Part model, mm, in its own coordinate system. A direction names the side the tool comes from. Round coordinates to 2 decimals unless told otherwise and drop trailing zeros. Loops run counter-clockwise (first coordinate to the right, second up) from the corner with the lowest first, then second, coordinate; pieces in that order, holes last. Notation, with made-up numbers: (40, 51) - (78, 51) arc R20 ccw to (78, 90) - close; hole circle Ø8 at (-4.5, 46.25). An arc over 180 degrees is marked (long way). Write each question's results on one line, items separated by ' | '. Start each with the question number.
(1) Cut at A-A, the plane z = 10. List the corners of the cut face in (x, y), then the cut area to 3 significant figures.
(2) Cut at D-D, the plane x = 2. List the corners of the cut face in (y, z), then the cut area to 3 significant figures.
(3) Mould opens along X. For faces 1 (the face through (0.14, -7.57, 19.4)), 2 (the face through (-1.06, 2.57, -18.48)), 3 (the face through (-10, -7.4, -5.8)) say: released by +X, released by -X, zero draft, split by the parting line, or undercut.
(4) Drill centre lines: L1, parallel to X at y = -9.4, z = -10; L2, parallel to Y at x = -3.5, z = 14. Where is each one in solid material? Low to high.
(5) Tool access for faces 4 (the face through (0, 3, -17)), 5 (the face through (0.1, 10, -19.5)): list every direction of +Z, -Z, +X, -X, +Y, -Y with a clear straight run to the whole face (end or side of a thin tool).
(6) Cut at C-C, the plane x = -3.25. List the corners of the cut face in (y, z).
(7) Cut at B-B, the plane y = 0. List the corners of the cut face in (x, z), then the cut area to 3 significant figures.
(8) Flat gauge pins, fed straight in: P1, Ø1.5, axis at x = 5, y = 2.5, coming from the +Z side; P2, Ø1.5, axis at x = -0.5, z = 15.5, coming from the +Y side. Where does each tip first touch, or does it go through?
from build123d import *

# Parameters (mm, degrees)
BOSS_EXTRUDE1_DEPTH     = 10
CUT_EXTRUDE1_DEPTH      = 43.426406871
CUT_EXTRUDE1_DEPTH_BACK = 43.426406871
SKETCH2_R               = 2.78
CUT_EXTRUDE2_DEPTH      = 31
CUT_EXTRUDE2_DEPTH_BACK = 31
SKETCH3_R               = 2.78


with BuildPart() as part:
    # Sketch1 → Boss-Extrude1 (new, symmetric)
    with BuildSketch(Plane(origin=(0, 0, 0), x_dir=(0, 0, -1), z_dir=(1, 0, 0))):
        with BuildLine():
            Line((-20, -10), (20, -10))
            Line((20, -10), (20, 10))
            Line((20, 10), (19, 10))
            ThreePointArc((19, 10), (17.585786438, 9.414213562), (17, 8))
            Line((17, 8), (17, -5))
            ThreePointArc((17, -5), (16.414213562, -6.414213562), (15, -7))
            Line((15, -7), (-18, -7))
            ThreePointArc((-18, -7), (-19.414213562, -7.585786438), (-20, -9))
            Line((-20, -9), (-20, -10))
        make_face()
    extrude(amount=BOSS_EXTRUDE1_DEPTH, both=True)

    # Sketch2 → Cut-Extrude1 (cut, two sides: drawn at the far end of the back side and taken through both)
    with BuildSketch(Plane(origin=(0, 0, -20), x_dir=(-1, 0, 0), z_dir=(0, 0, -1)).offset(-CUT_EXTRUDE1_DEPTH_BACK)):
        with Locations(Location((0, 0, 0), (0, 0, 90))):
            Circle(SKETCH2_R)
    extrude(amount=CUT_EXTRUDE1_DEPTH + CUT_EXTRUDE1_DEPTH_BACK, mode=Mode.SUBTRACT)

    # Sketch3 → Cut-Extrude2 (cut, two sides: drawn at the far end of the back side and taken through both)
    with BuildSketch(Plane.XZ.offset(10).offset(-CUT_EXTRUDE2_DEPTH_BACK)):
        with Locations(Location((0, 10, 0), (0, 0, 270))):
            Circle(SKETCH3_R)
        with Locations(Location((0, -10, 0), (0, 0, 270))):
            Circle(SKETCH3_R)
    extrude(amount=CUT_EXTRUDE2_DEPTH + CUT_EXTRUDE2_DEPTH_BACK, mode=Mode.SUBTRACT)


solid = part.part
A:
1) outline: (-10, -10) - (-2.78, -10) - (-2.78, -7) - (-10, -7) - close; (2.78, -10) - (10, -10) - (10, -7) - (2.78, -7) - close | area: 43.3 mm2
2) outline: (-10, -20) - (-1.93, -20) - (-1.93, -17) - (-5, -17) arc R2 cw to (-7, -15) - (-7, -11.93) - (-10, -11.93) - close; (-10, -8.07) - (-7, -8.07) - (-7, 8.07) - (-10, 8.07) - close; (-10, 11.93) - (-7, 11.93) - (-7, 18) arc R2 ccw to (-9, 20) - (-10, 20) - close; (1.93, -20) - (10, -20) - (10, -19) arc R2 ccw to (8, -17) - (1.93, -17) - close | area: 135 mm2
3) face 1: zero draft | face 2: undercut | face 3: released by -X
4) L1: -10 to -2.78, 2.78 to 10 | L2: -10 to -7
5) face 4: +Z, +X, -X, +Y | face 5: +Z, -Z, +X, -X, +Y
6) outline: (-10, -20) - (10, -20) - (10, -19) arc R2 ccw to (8, -17) - (-5, -17) arc R2 cw to (-7, -15) - (-7, 18) arc R2 ccw to (-9, 20) - (-10, 20) - close
7) outline: (-10, -20) - (-2.78, -20) - (-2.78, -17) - (-10, -17) - close; (2.78, -20) - (10, -20) - (10, -17) - (2.78, -17) - close | area: 43.3 mm2
8) P1: z = -17 | P2: y = -7
